The figure shows three views and two pictorial views of one solid part (mm, origin at its lowest corner). Answer the questions. A direction names the side the tool comes from. Round coordinates to 2 decimals unless told otherwise and drop trailing zeros. Order: outer loops, then holes, each group sorted by start corner. A loop starts at its lowest first (then second) coordinate and runs counter-clockwise, first axis right, second up. Notation, with made-up numbers: (89.25, 56) -> (141.25, 56) arc R25 cw to (141.25, 69) -> close; hole circle Ø5 at (23.5, 71). An arc over 180 degrees is marked (long way). Answer in a Markdown table with one row per item. Add a question column.
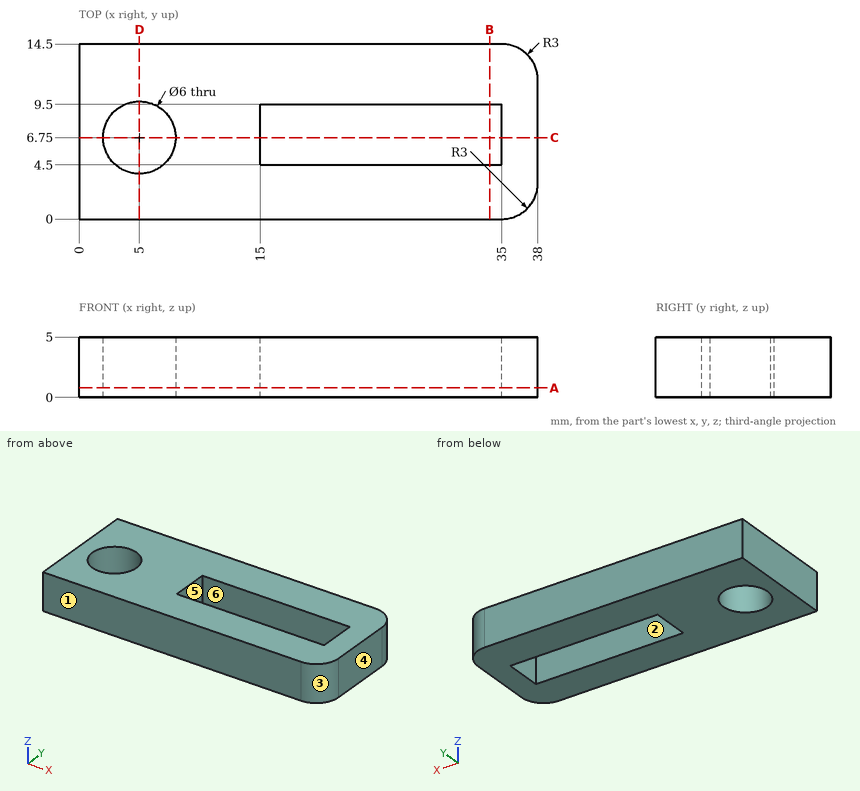
1. The part is cut by section B-B (x = 34). Give the vertices of the cut face in (y, z).
2. Straight lines are drawn through the part: line 1 along Y through (x, z) = (5, 1.95); line 2 along Y through (x, z) = (17.5, 4.15); line 3 along X through (y, z) = (5, 4.25). For each, find the intervals that lie inside material, in ascending order.
3. The part is cut by section C-C (y = 6.75). Give the vertices of the cut face in (x, z).
4. The part is cut by section D-D (x = 5). Give the vertices of the cut face in (y, z), then the cut area to 3 significant figures.
5. This flat-tipped pin is pushed along its axis until it touches: pin 1 (1.5 mm diameter, centred on x = 34, y = 12.5, fed in from -Z). Where does it stop, or does it pass through?
6. The mould has two halves that part along Y. Classify the marked faces 3, 4, 5 and 6: released by +Y, released by -Y, zero draft, split by the parting line, or undercut.
7. For the marked faces 1 and 2, determine the directions among +Z, -Z, +X, -X, +Y, -Y from which every point of the face is accessible in a straight line to the end or side of a thin tool.
8. The part is cut by section A-A (z = 0.8). Give the vertices of the cut face in (x, y), then the cut area to 3 significant figures.
Report:
| question | item | result |
|---|---|---|
| 1 | outline | (0, 0) -> (4.5, 0) -> (4.5, 5) -> (0, 5) -> close; (9.5, 0) -> (14.5, 0) -> (14.5, 5) -> (9.5, 5) -> close |
| 2 | line 1 | y = 0 to 3.75, 9.75 to 14.5 |
| 2 | line 2 | y = 0 to 4.5, 9.5 to 14.5 |
| 2 | line 3 | x = 0 to 2.56, 7.44 to 15, 35 to 38 |
| 3 | outline | (0, 0) -> (2, 0) -> (2, 5) -> (0, 5) -> close; (8, 0) -> (15, 0) -> (15, 5) -> (8, 5) -> close; (35, 0) -> (38, 0) -> (38, 5) -> (35, 5) -> close |
| 4 | outline | (0, 0) -> (3.75, 0) -> (3.75, 5) -> (0, 5) -> close; (9.75, 0) -> (14.5, 0) -> (14.5, 5) -> (9.75, 5) -> close |
| 4 | area | 42.5 mm^2 |
| 5 | pin 1 | stops at z = 0 |
| 6 | face 3 | released by -Y |
| 6 | face 4 | zero draft |
| 6 | face 5 | undercut |
| 6 | face 6 | undercut |
| 7 | face 1 | +Z, -Z, +X, -X, -Y |
| 7 | face 2 | +Z, -Z |
| 8 | outline | (0, 0) -> (35, 0) arc R3 ccw to (38, 3) -> (38, 11.5) arc R3 ccw to (35, 14.5) -> (0, 14.5) -> close; hole circle Ø6 at (5, 6.75); hole (15, 4.5) -> (35, 4.5) -> (35, 9.5) -> (15, 9.5) -> close |
| 8 | area | 419 mm^2 |
